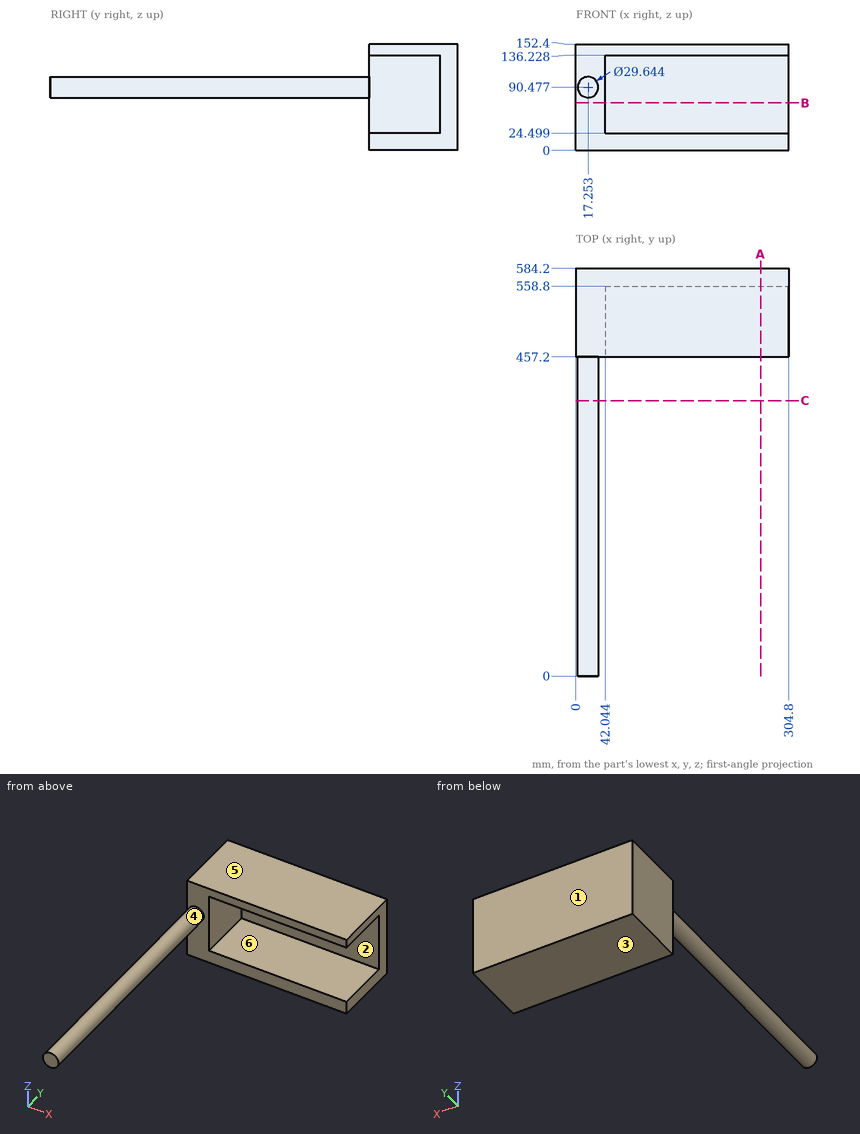
For this review, use the dimensioned drawing (mm, ordinates from the lowest corner) and the shaded views. A direction names the side the tool comes from. Give positions to 0.01 mm unless a question says otherwise; leave off trailing zeros. Write each loop counter-clockwise with the first axis right and the second up, starting at its lowest first coordinate (ties: lowest second). Pieces come first, ordered by that corner, then holes. Notation, with made-up numbers: M -6,59 L 44,59 A21 cw 44,72 Z; hole C 85,-5 d11. An arc over 180 degrees is marked long. Answer as a JSON object with one key per item and string values. Group by question number.
1) Mouldability with a two-part tool opening along Z and no side actions: class the marked faces 1, 2 and 3 as released by +Z, released by -Z, zero draft, split by the parting line, or undercut.
2) We need section A-A (x = 264.5). Give the boundary of the cut face in (y, z).
3) We need section C-C (y = 394.5). Give the boundary of the cut face in (x, z) (1 decimal).
4) We need section B-B (z = 68). Give the boundary of the cut face in (x, y).
5) For line 1 along Z through (x, y) = (255, 500.5); line 2 along Y through (x, z) = (144.5, 88.5); line 3 along X through (y, z) = (522, 72), list the stretches that pass through material, from the lowest coordinate up.
6) Tool access review of the marked faces 4, 5 and 6: name each direction out of +Z, -Z, +X, -X, +Y, -Y from which nothing blocks a thin tool from reaching the whole face with its end or side.
7) Clearance check with flat-ended pins moving along their axes: pin 1 Ø1.5 at (x, y) = (273, 472.5) entering from -Z; pin 2 Ø12 at (x, z) = (145, 65.5) entering from -Y; pin 3 Ø6 at (y, z) = (252.5, 101) entering from +X (1 decimal). State where each tip first meets the part, or that it passes through.
Answer key:
{
 "1": {"face 1": "zero draft", "face 2": "undercut", "face 3": "released by -Z"},
 "2": {"outline": "M 457.2,0 L 584.2,0 L 584.2,152.4 L 457.2,152.4 L 457.2,136.23 L 558.8,136.23 L 558.8,24.5 L 457.2,24.5 Z"},
 "3": {"outline": "C 17.3,90.5 d29.6"},
 "4": {"outline": "M 0,457.2 L 42.04,457.2 L 42.04,558.8 L 304.8,558.8 L 304.8,584.2 L 0,584.2 Z"},
 "5": {"line 1": "z = 0 to 24.5, 136.23 to 152.4", "line 2": "y = 558.8 to 584.2", "line 3": "x = 0 to 42.04"},
 "6": {"face 4": "-Y", "face 5": "+Z, +X, -X, +Y, -Y", "face 6": "+X, -Y"},
 "7": {"pin 1": "stops at z = 0", "pin 2": "stops at y = 558.8", "pin 3": "stops at x = 30"}
}
